The listing builds one solid part. Answer for the finished solid, in the listing's coordinates (mm). Face numbers are marked on the shaded views. A direction names the side the tool comes from. Round coordinates to 2 decimals unless told otherwise and drop trailing zeros. Write each loop counter-clockwise with the first axis right and the second up, starting at its lowest first coordinate (ties: lowest second). Pieces come first, ordered by that corner, then holes. Notation, with made-up numbers: (67.25, 29) -> (72.25, 29) arc R28 ccw to (72.25, 63) -> close; hole circle Ø4 at (-1, -24.5). An arc over 180 degrees is marked (long way). Write each question's results on one line, items separated by ' | '. Start each with the question number.
```python
from build123d import *

# Parameters (mm, degrees)
BOSS_EXTRUDE1_DEPTH = 47
CUT_EXTRUDE1_REACH  = 57.376
SKETCH2_R           = 1.75


with BuildPart() as part:
    # Sketch1 → Boss-Extrude1 (new body)
    with BuildSketch(Plane(origin=(0, 0, 0), x_dir=(0, 1, 0), z_dir=(0, 0, 1))):
        with BuildLine():
            Line((1, 12.760877713), (1, 26.8))
            Line((1, 26.8), (5, 26.8))
            Line((5, 26.8), (5, 16.038703189))
            ThreePointArc((5, 16.038703189), (16.8, 0), (5, -16.038703189))
            Line((5, -16.038703189), (5, -26.8))
            Line((5, -26.8), (1, -26.8))
            Line((1, -26.8), (1, -12.760877713))
            ThreePointArc((1, -12.760877713), (12.8, 0), (1, 12.760877713))
        make_face()
    extrude(amount=BOSS_EXTRUDE1_DEPTH)

    # Sketch2 → Cut-Extrude1 (cut, up to next)
    with BuildSketch(Plane(origin=(0, 5, 0), x_dir=(-1, 0, 0), z_dir=(0, 1, 0)), mode=Mode.PRIVATE) as cut_extrude1_sk1:
        with Locations((-21.8, 40)):
            Circle(SKETCH2_R)
    cut_extrude1_tool1 = extrude(cut_extrude1_sk1.sketch, amount=-CUT_EXTRUDE1_REACH, mode=Mode.PRIVATE) & part.part
    # Sketch2 → Cut-Extrude1 (cut, up to next)
    with BuildSketch(Plane(origin=(0, 5, 0), x_dir=(-1, 0, 0), z_dir=(0, 1, 0)), mode=Mode.PRIVATE) as cut_extrude1_sk2:
        with Locations((-21.8, 7)):
            Circle(SKETCH2_R)
    cut_extrude1_tool2 = extrude(cut_extrude1_sk2.sketch, amount=-CUT_EXTRUDE1_REACH, mode=Mode.PRIVATE) & part.part
    # Sketch2 → Cut-Extrude1 (cut, up to next)
    with BuildSketch(Plane(origin=(0, 5, 0), x_dir=(-1, 0, 0), z_dir=(0, 1, 0)), mode=Mode.PRIVATE) as cut_extrude1_sk3:
        with Locations((21.8, 7)):
            Circle(SKETCH2_R)
    cut_extrude1_tool3 = extrude(cut_extrude1_sk3.sketch, amount=-CUT_EXTRUDE1_REACH, mode=Mode.PRIVATE) & part.part
    # Sketch2 → Cut-Extrude1 (cut, up to next)
    with BuildSketch(Plane(origin=(0, 5, 0), x_dir=(-1, 0, 0), z_dir=(0, 1, 0)), mode=Mode.PRIVATE) as cut_extrude1_sk4:
        with Locations((21.8, 40)):
            Circle(SKETCH2_R)
    cut_extrude1_tool4 = extrude(cut_extrude1_sk4.sketch, amount=-CUT_EXTRUDE1_REACH, mode=Mode.PRIVATE) & part.part
    add(cut_extrude1_tool1.solids().sort_by_distance((21.8, 5, 40))[0], mode=Mode.SUBTRACT)
    add(cut_extrude1_tool2.solids().sort_by_distance((21.8, 5, 7))[0], mode=Mode.SUBTRACT)
    add(cut_extrude1_tool3.solids().sort_by_distance((-21.8, 5, 7))[0], mode=Mode.SUBTRACT)
    add(cut_extrude1_tool4.solids().sort_by_distance((-21.8, 5, 40))[0], mode=Mode.SUBTRACT)


solid = part.part
```
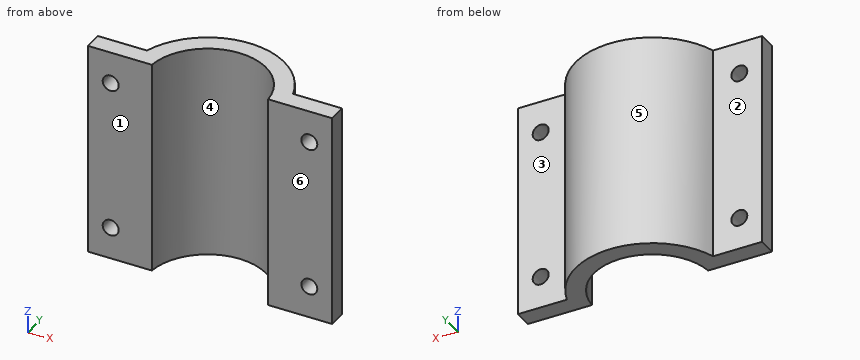
Q1. Each of these flat-tipped pins is pushed along its axis until it touches: pin 1 (2 mm diameter, centred on x = 16.5, y = 8.5, fed in from -Z); pin 2 (1.5 mm diameter, centred on y = 14.5, z = 7, fed in from +X); pin 3 (1 mm diameter, centred on x = -15.5, z = 39, fed in from +Y); pin 4 (12 mm diameter, centred on x = 20, z = 15, fed in from +Y). Where does it stop, or does it pass through?
Q2. The part is cut by section C-C, the plane y = 3. Write down the section's boundary in (x, z), then the cut area to 3 significant figures.
Q3. The part is cut by section B-B, the plane z = 40. Write down the section's boundary in (x, y), then the cut area to 3 significant figures.
Q4. The part is cut by section A-A, the plane x = 21.8. Write down the section's boundary in (y, z), then the cut area to 3 significant figures.
Q5. Find the intervals of material crossed by line 1 (Z direction, x = -21.8, y = 4.25); line 2 (Y direction, x = -21.5, z = 29.5); line 3 (Y direction, x = -0.5, z = 38.5), in increasing order.
Q6. The part is cut by section D-D, the plane y = 10. Write down the section's boundary in (x, z).
Q7. Determine the mould class of the marked faces 4, 5 and 6 for opening direction X: pulls with the +X half, pulls with the -X half, needs draft (parallel to the pull), parting line crosses it, or undercut.
Q8. For the marked faces 1, 2 and 3, determine the directions among +Z, -Z, +X, -X, +Y, -Y from which every point of the face is accessible in a straight line to the end or side of a thin tool.
Answers follow:
1) pin 1: through | pin 2: x = 9.65 | pin 3: y = 7.57 | pin 4: y = 9.29
2) outline: (-26.8, 0) -> (-12.44, 0) -> (-12.44, 47) -> (-26.8, 47) -> close; (12.44, 0) -> (26.8, 0) -> (26.8, 47) -> (12.44, 47) -> close; hole circle Ø3.5 at (-21.8, 7); hole circle Ø3.5 at (-21.8, 40); hole circle Ø3.5 at (21.8, 7); hole circle Ø3.5 at (21.8, 40) | area: 1,310 mm^2
3) outline: (-26.8, 1) -> (-23.55, 1) -> (-23.55, 5) -> (-26.8, 5) -> close; (-20.05, 1) -> (-12.76, 1) arc R12.8 cw to (12.76, 1) -> (20.05, 1) -> (20.05, 5) -> (16.04, 5) arc R16.8 ccw to (-16.04, 5) -> (-20.05, 5) -> close; (23.55, 1) -> (26.8, 1) -> (26.8, 5) -> (23.55, 5) -> close | area: 232 mm^2
4) outline: (1, 0) -> (5, 0) -> (5, 5.25) -> (1, 5.25) -> close; (1, 8.75) -> (5, 8.75) -> (5, 38.25) -> (1, 38.25) -> close; (1, 41.75) -> (5, 41.75) -> (5, 47) -> (1, 47) -> close | area: 160 mm^2
5) line 1: 0 to 5.25, 8.75 to 38.25, 41.75 to 47 | line 2: 1 to 5 | line 3: 12.79 to 16.79
6) outline: (-13.5, 0) -> (-7.99, 0) -> (-7.99, 47) -> (-13.5, 47) -> close; (7.99, 0) -> (13.5, 0) -> (13.5, 47) -> (7.99, 47) -> close
7) face 4: undercut | face 5: parting line crosses it | face 6: needs draft
8) face 1: +Z, -Z, +X, -X, -Y | face 2: +Z, -Z, -X, +Y | face 3: +Z, -Z, +X, +Y
